Could you check a few things on this drawing? It's one solid part, dimensions in mm from its lowest x, y, z. A direction names the side the tool comes from. Coordinates: 2 decimals unless noted, no trailing zeros. Loops run counter-clockwise (first coordinate to the right, second up) from the corner with the lowest first, then second, coordinate; pieces in that order, holes last. Notation, with made-up numbers: (83, 81) -> (126, 81) arc R21 cw to (126, 91) -> close; hole circle Ø1 at (69.5, 24). An arc over 180 degrees is marked (long way). One line per question, with ' | ' between items.
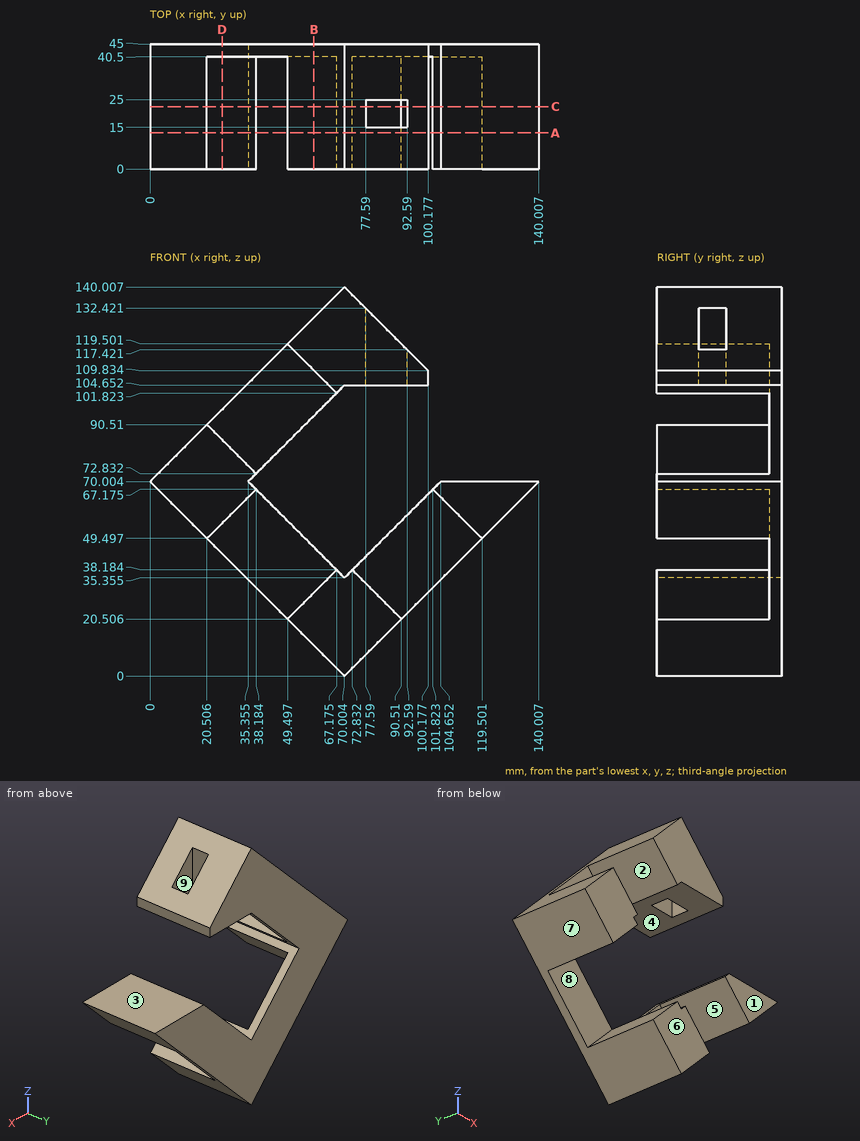
1) I'm going to push flat-ended pins straight in: pin 1 Ø17.5 at (x, y) = (116, 12) entering from +Z; pin 2 Ø3 at (y, z) = (18, 120) entering from +X; pin 3 Ø4 at (x, y) = (114.5, 7) entering from -Z; pin 4 Ø5 at (x, z) = (124.5, 50.5) entering from -Y. Where does each tip first touch, or does it pass through?
Data:
pin 1: z = 70 | pin 2: x = 77.59 | pin 3: z = 52.5 | pin 4: through
2) On a 3-axis mill with a long thin cutter (end or side, diameter ignored), from which of +Z, -Z, +X, -X, +Y, -Y can I reach the whole of each face in a straight line? I mean the marked faces 1, 2, 3, 4 and 5. Say none if no direction works.
Data:
face 1: +Z, -Z, +X, -X, -Y | face 2: -X, -Y | face 3: +Z, +X, +Y, -Y | face 4: +X, +Y, -Y | face 5: -Z, -Y
3) If we section it at B-B on x = 59: Please give me the cut outline in (y, z).
Data:
outline: (0, 11) -> (45, 11) -> (45, 46.36) -> (40.5, 46.36) -> (40.5, 30.01) -> (0, 30.01) -> close; (0, 110) -> (40.5, 110) -> (40.5, 93.65) -> (45, 93.65) -> (45, 129) -> (0, 129) -> close
4) If we section it at C-C on y = 22.5: Please give me the cut outline in (x, z) (1 decimal), and give its area (3 significant figures).
Data:
outline: (0, 70) -> (20.5, 49.5) -> (38.2, 67.2) -> (35.4, 70) -> (38.2, 72.8) -> (20.5, 90.5) -> close; (49.5, 20.5) -> (70, 0) -> (90.5, 20.5) -> (72.8, 38.2) -> (70, 35.4) -> (67.2, 38.2) -> close; (49.5, 119.5) -> (67.2, 101.8) -> (70, 104.7) -> (77.6, 104.7) -> (77.6, 132.4) -> (70, 140) -> close; (92.6, 104.7) -> (100.2, 104.7) -> (100.2, 109.8) -> (92.6, 117.4) -> close; (101.8, 67.2) -> (119.5, 49.5) -> (140, 70) -> (104.7, 70) -> close | area: 2,780 mm²
5) I need wall thicknesses on line 1 along Y through (x, z) = (60, 98); line 2 along Z through (x, y) = (59, 31.5) (1 decimal); line 3 along X through (y, z) = (2.5, 56) (1 decimal). Which ranges of each line are inside material? Lowest first, please. Write a range as from..to.
Data:
line 1: 40.5..45 | line 2: 11..30, 110..129 | line 3: 14..27, 113..126
6) If we section it at D-D on x = 26: Please give me the cut outline in (y, z) (1 decimal).
Data:
outline: (0, 55) -> (40.5, 55) -> (40.5, 44) -> (45, 44) -> (45, 96) -> (40.5, 96) -> (40.5, 85) -> (0, 85) -> close
7) If we section it at A-A on y = 13: Please give me the cut outline in (x, z) (1 decimal), and give its area (3 significant figures).
Data:
outline: (0, 70) -> (20.5, 49.5) -> (38.2, 67.2) -> (35.4, 70) -> (38.2, 72.8) -> (20.5, 90.5) -> close; (49.5, 20.5) -> (70, 0) -> (90.5, 20.5) -> (72.8, 38.2) -> (70, 35.4) -> (67.2, 38.2) -> close; (49.5, 119.5) -> (67.2, 101.8) -> (70, 104.7) -> (100.2, 104.7) -> (100.2, 109.8) -> (70, 140) -> close; (101.8, 67.2) -> (119.5, 49.5) -> (140, 70) -> (104.7, 70) -> close | area: 3,090 mm²
8) We'd pull the mould along X, two halves only. Please class the marked faces 6, 7, 8 and 9: pulls with the +X half, pulls with the -X half, needs draft (parallel to the pull), parting line crosses it, or undercut.
Data:
face 6: needs draft | face 7: pulls with the -X half | face 8: undercut | face 9: undercut
